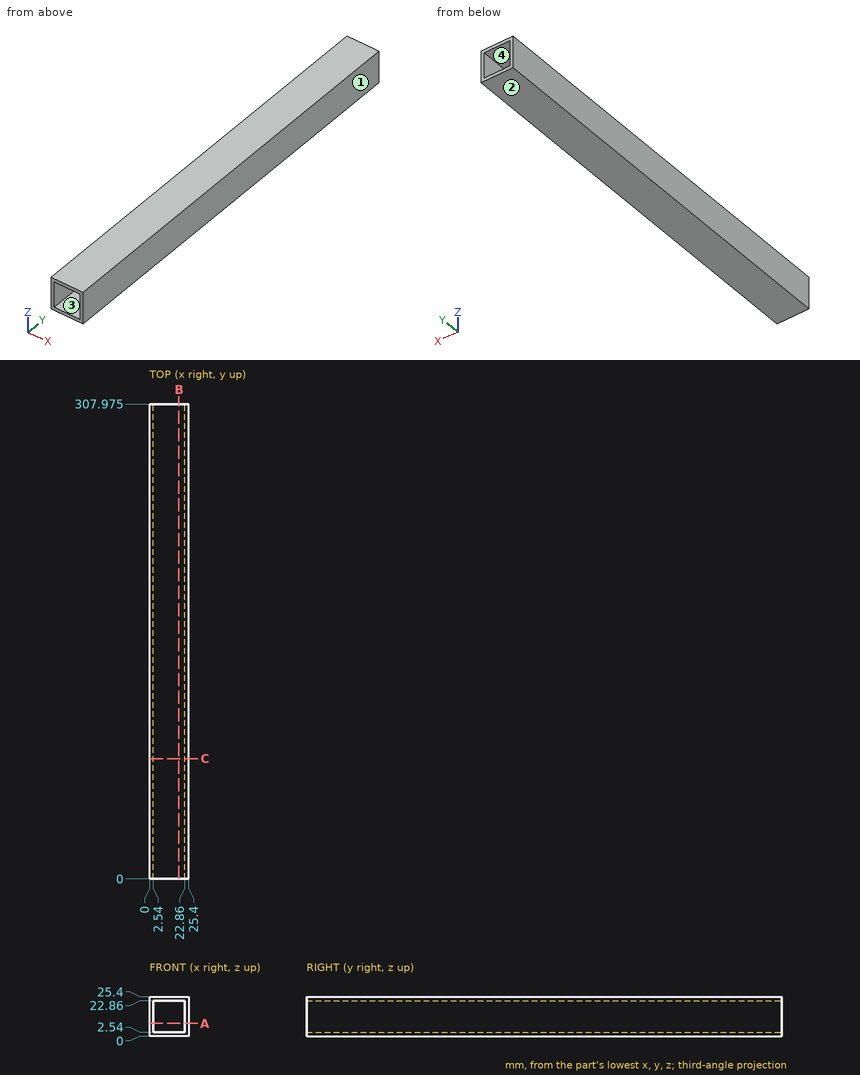
Print and shaded views of the part. All mm, measured from the part's lowest x, y and z. Round coordinates to 2 decimals unless told otherwise and drop trailing zeros. Order: outer loops, then holes, each group sorted by start corner. A loop starts at its lowest first (then second) coordinate and runs counter-clockwise, first axis right, second up. Notation, with made-up numbers: (53, 1) - (75, 1) arc R21 cw to (75, 7) - close; hole circle Ø8 at (73, 6). An arc over 180 degrees is marked (long way). Use a Markdown table: item, result.
1) Saw through at B-B on x = 19. Write the cut outline in (y, z) (3 decimals).
Recorded:
| item | result |
|---|---|
| outline | (0, 0) - (307.975, 0) - (307.975, 2.54) - (0, 2.54) - close; (0, 22.86) - (307.975, 22.86) - (307.975, 25.4) - (0, 25.4) - close |
2) Saw through at C-C on y = 78. Write the cut outline in (x, z), and give its area (3 significant figures).
Recorded:
| item | result |
|---|---|
| outline | (0, 0) - (25.4, 0) - (25.4, 25.4) - (0, 25.4) - close; hole (2.54, 2.54) - (22.86, 2.54) - (22.86, 22.86) - (2.54, 22.86) - close |
| area | 232 mm² |
3) Saw through at A-A on z = 8.25. Write the cut outline in (x, y) (3 decimals), and give its area (3 significant figures).
Recorded:
| item | result |
|---|---|
| outline | (0, 0) - (2.54, 0) - (2.54, 307.975) - (0, 307.975) - close; (22.86, 0) - (25.4, 0) - (25.4, 307.975) - (22.86, 307.975) - close |
| area | 1,560 mm² |
4) Pull direction Z, two halves, no side cores. Call the marked faces 1, 2, 3 and 4: pulls with the +Z half, pulls with the -Z half, needs draft (parallel to the pull), parting line crosses it, or undercut.
Recorded:
| item | result |
|---|---|
| face 1 | needs draft |
| face 2 | pulls with the -Z half |
| face 3 | undercut |
| face 4 | undercut |
5) Wall check: L1, parallel to Z at x = 20, y = 213.5. Give the ranges that are in metal, low to high.
Recorded:
| item | result |
|---|---|
| L1 | z = 0 to 2.54, 22.86 to 25.4 |
